```python
from build123d import *

# Parameters (mm, degrees)
F1_DEPTH     = 75
F2_T         = -3
F3_SIZE      = 5
F4_T1_DEPTH  = 60.9562282093
F4_T3_DEPTH  = 60.9562282093
F4_T5_DEPTH  = 60.9562282093
F4_T7_DEPTH  = 60.9562282093
F4_T9_DEPTH  = 60.9562282093
F4_T11_DEPTH = 60.9562282093
F6_D         = 10
F7_T1_DEPTH  = 80.3079500043


# Not quite as in the source:
# - a fillet or chamfer that OpenCascade refuses, or shapes differently, is made with other operations: its cross-section is extruded or revolved along the edge and cut away or added


with BuildPart() as f1:
    # F0 (on Top) → F1 (new body)
    with BuildSketch(Plane.XY):
        Polygon((-0.2972451442, 35.2381446725), (-30.6657510407, 17.3616504902), (-30.3685058965, -17.8764941822), (0.2972451442, -35.2381446725), (30.6657510407, -17.3616504902), (30.3685058965, 17.8764941822), align=None)
    extrude(amount=F1_DEPTH)

    # F2
    f2_openings = [f1.faces().sort_by_distance(p)[0] for p in [
        (0, 0, 75),
    ]]
    offset(amount=F2_T, openings=f2_openings)

    # F3
    f3_edges = [f1.edges().sort_by_distance(p)[0] for p in [
        (15.03563, 26.557319, 0),
        (-15.481498, 26.299898, 0),
        (-30.517128, -0.257422, 0),
        (-15.03563, -26.557319, 0),
        (15.481498, -26.299898, 0),
        (30.517128, 0.257422, 0),
    ]]
    chamfer(f3_edges, length=F3_SIZE)

    # F4: chamfer of 5 on 6 edges, made by hand

    # F4_s2 → F4_t1 (cut)
    with BuildSketch(Plane(origin=(-26.5224238672, 15.0158739867, 0), x_dir=(0, 0, 1), z_dir=(0.8702121062, -0.4926772679, 0))):
        Polygon((75, 25.5182141675), (70, 30.5182141675), (75, 30.5182141675), align=None)
    extrude(amount=F4_T1_DEPTH, mode=Mode.SUBTRACT)

    # F4_s4 → F4_t3 (cut)
    with BuildSketch(Plane(origin=(-0.257083601, 30.4770298323, 0), x_dir=(0, 0, 1), z_dir=(0.0084350232, -0.9999644246, 0))):
        Polygon((75, 25.5182141675), (70, 30.5182141675), (75, 30.5182141675), align=None)
    extrude(amount=F4_T3_DEPTH, mode=Mode.SUBTRACT)

    # F4_s6 → F4_t5 (cut)
    with BuildSketch(Plane(origin=(26.2653402661, 15.4611558455, 0), x_dir=(0, 0, 1), z_dir=(-0.8617770829, -0.5072871567, 0))):
        Polygon((75, 25.5182141675), (70, 30.5182141675), (75, 30.5182141675), align=None)
    extrude(amount=F4_T5_DEPTH, mode=Mode.SUBTRACT)

    # F4_s8 → F4_t7 (cut)
    with BuildSketch(Plane(origin=(26.5224238672, -15.0158739867, 0), x_dir=(0, 0, 1), z_dir=(-0.8702121062, 0.4926772679, 0))):
        Polygon((70, 30.5182141675), (75, 25.5182141675), (75, 30.5182141675), align=None)
    extrude(amount=F4_T7_DEPTH, mode=Mode.SUBTRACT)

    # F4_s10 → F4_t9 (cut)
    with BuildSketch(Plane(origin=(0.257083601, -30.4770298323, 0), x_dir=(0, 0, 1), z_dir=(-0.0084350232, 0.9999644246, 0))):
        Polygon((70, 30.5182141675), (75, 25.5182141675), (75, 30.5182141675), align=None)
    extrude(amount=F4_T9_DEPTH, mode=Mode.SUBTRACT)

    # F4_s12 → F4_t11 (cut)
    with BuildSketch(Plane(origin=(-26.2653402661, -15.4611558455, 0), x_dir=(0, 0, 1), z_dir=(0.8617770829, 0.5072871567, 0))):
        Polygon((75, 25.5182141675), (70, 30.5182141675), (75, 30.5182141675), align=None)
    extrude(amount=F4_T11_DEPTH, mode=Mode.SUBTRACT)

    # F6 (through all)
    with Locations(Plane(origin=(-15.0356303762, -26.5573194273, 0), x_dir=(0.8702121062, -0.4926772679, 0), z_dir=(-0.4926772679, -0.8702121062, 0))):
        with Locations((0, 52.5516085327)):
            Hole(F6_D / 2)

    # F7: chamfer of 5 on 8 edges, made by hand

    # F7_s2 → F7_t1 (cut)
    with BuildSketch(Plane.XY.offset(-2.6539750021)):
        Polygon((-30.3928557112, -14.9898455337), (-27.8564199277, -19.2987309484), (-30.3685058965, -17.8764941822), align=None)
        Polygon((-28.1780148866, 18.8260623726), (-30.6414012259, 14.4750018417), (-30.6657510407, 17.3616504902), align=None)
        Polygon((2.2148408246, 33.8159079063), (-2.7849812982, 33.7737327901), (-0.2972451442, 35.2381446725), align=None)
        Polygon((27.8564199277, 19.2987309484), (30.3928557112, 14.9898455337), (30.3685058965, 17.8764941822), align=None)
        Polygon((30.6414012259, -14.4750018417), (28.1780148866, -18.8260623726), (30.6657510407, -17.3616504902), align=None)
        Polygon((2.7849812982, -33.7737327901), (-2.2148408246, -33.8159079063), (0.2972451442, -35.2381446725), align=None)
    extrude(amount=F7_T1_DEPTH, mode=Mode.SUBTRACT)

    # F7_s3 → F7_t4 (revolve, cut)
    with BuildSketch(Plane.XY.offset(52.5516085327)):
        Polygon((23.7377514379, 21.6305467487), (16.9233045677, 19.7428725572), (19.386690907, 24.093933088), align=None)
    revolve(axis=Axis((15.0356303762, 26.5573194273, 52.5516085327), (-0.4926772679, -0.8702121062, 0)), mode=Mode.SUBTRACT)

    # F7_s5 → F7_t6 (revolve, cut)
    with BuildSketch(Plane.XY.offset(52.5516085327)):
        Polygon((-6.3335093144, -31.484092106), (-8.221183506, -24.6696452358), (-10.6845698453, -29.0207057667), align=None)
    revolve(axis=Axis((-15.0356303762, -26.5573194273, 52.5516085327), (-0.4926772679, -0.8702121062, 0)), mode=Mode.SUBTRACT)


solid = f1.part
```
For this review, take the finished solid that the model builds, in its own axes (mm). A direction names the side the tool comes from. Give positions to 0.01 mm unless a question says otherwise; leave off trailing zeros. Loops run counter-clockwise (first coordinate to the right, second up) from the corner with the lowest first, then second, coordinate; pieces in that order, holes last. Notation, with made-up numbers: M 29,67 L 76,67 A17 ccw 76,97 Z; hole C -31,43 d8. An arc over 180 degrees is marked long. One line per item, written item: value. Start each with the question number.
Q1. Add section B-B (y = 0). Give the boundary of the cut face in (x, z).
Q2. Add section A-A (z = 10.5). Give the boundary of the cut face in (x, y) (3 decimals), and give its area (3 significant figures).
Q3. For L1, parallel to Z at x = 11.5, y = 11.5; L2, parallel to X at y = 17, z = 19; L3, parallel to X at y = 20, z = 26.5, list the stretches that pass through material, from the lowest coordinate up.
Q4. Machinability: for faces 1 (the face through (-29.142, -17.114, 37.028)), 2 (the face through (-13.75, -23.84, 37.51)), which of the approach directions +Z, -Z, +X, -X, +Y, -Y give a long, thin tool a straight path to every point of the face, cutting with its end or side? Answer none if there is none.
Q5. Clearance check with flat-ended pins moving along their axes: pin 1 Ø4 at (x, z) = (-23.5, 65.5) entering from +Y; pin 2 Ø6 at (y, z) = (26, 41.5) entering from -X; pin 3 Ø1 at (x, z) = (22, 26.5) entering from -Y. State where each tip first meets the part, or that it passes through.
Reply:
1. outline: M -30.52,5 L -25.52,0 L 25.52,0 L 30.52,5 L 30.52,70 L 27.52,73 L 27.52,3 L -27.52,3 L -27.52,73 L -30.52,70 Z
2. outline: M -30.641,14.475 L -30.393,-14.99 L -27.856,-19.299 L -2.215,-33.816 L 2.785,-33.774 L 28.178,-18.826 L 30.641,-14.475 L 30.393,14.99 L 27.856,19.299 L 2.215,33.816 L -2.785,33.774 L -28.178,18.826 Z; hole M -27.651,15.655 L -27.383,-16.119 L 0.268,-31.774 L 27.651,-15.655 L 27.383,16.119 L -0.268,31.774 Z
2. area: 581 mm²
3. L1: 0 to 3
3. L2: -29.21 to -25.37, 25.83 to 29.21
3. L3: -26.18 to -20.27, 20.53 to 26.62
4. face 1: +Z, -Z, -X, -Y
4. face 2: +Z
5. pin 1: y = 22.76
5. pin 2: x = -21.09
5. pin 3: y = -22.76
